Autodesk Inventor part; units mm, degrees
ref_plane "YZ Plane" through (0, 0, 0) normal (1, 0, 0) x (0, 1, 0)
ref_plane "XZ Plane" through (0, 0, 0) normal (0, 1, 0) x (-1, 0, 0)
ref_plane "XY Plane" through (0, 0, 0) normal (0, 0, 1) x (1, 0, 0)
sketch "Sketch1" plane through (0, 0, 0) normal (0, 0, 1) x (1, 0, 0)
  circle A0 centre (0, 0) radius 19.685
  dimension "d0" = 39.37
extrude "Extrusion1" add sketch "Sketch1" along normal blind 43.815
sketch "Sketch2" plane through (0, 0, 43.815) normal (0, 0, 1) x (1, 0, 0)
  circle A0 centre (0, 0) radius 19.685
  circle A1 centre (0, 0) radius 26.035
  dimension "d4" = 52.07
extrude "Extrusion2" add sketch "Sketch2" along normal blind 1.27 contours A0 | A1
fillet "Fillet1" radius 3.175 2 edges at (-19.685, 0, 0) (-19.685, 0, 43.815)
sketch "Sketch3" plane through (0, 0, 0) normal (0, 0, -1) x (-1, 0, 0)
  circle A0 centre (0, 0) radius 16.51
  circle A1 centre (0, 0) radius 3.175
  dimension "d9" = 6.35
extrude "Extrusion3" cut sketch "Sketch3" against normal blind 2.54 contours A1
properties part number "Lg Motor Top" material "ABS Plastic"
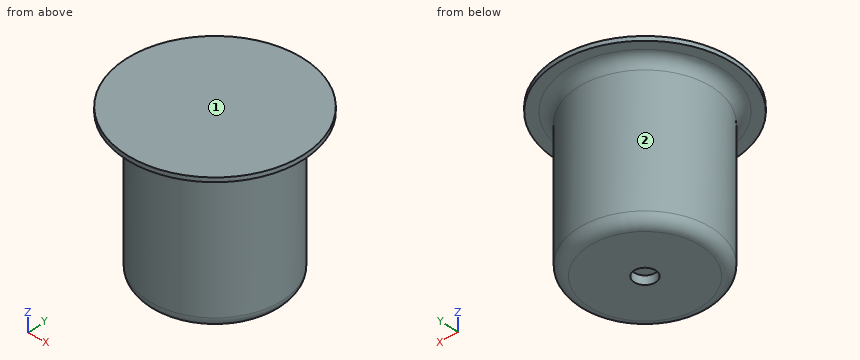
For this review, take the finished solid that the model builds, in its own axes (mm). Face numbers are marked on the shaded views. A direction names the side the tool comes from. Round coordinates to 2 decimals unless told otherwise and drop trailing zeros. Write each loop counter-clockwise with the first axis right and the second up, starting at its lowest first coordinate (ties: lowest second). Pieces come first, ordered by that corner, then holes. Notation, with made-up numbers: (3, 50) -> (20, 50) arc R30 cw to (20, 85) -> close; hole circle Ø11 at (22.5, 53). An arc over 180 degrees is marked (long way). One line per question, with ' | ' between items. Start each with the question number.
1) Add section A-A (x = 0). Write out the cut boundary in (y, z) (3 decimals).
2) For pin 1 Ø5 at (x, z) = (-0.5, 18.5) entering from -Y (3 decimals); pin 2 Ø10 at (x, y) = (-16.5, -15.5) entering from -Z; pin 3 Ø1 at (y, z) = (16.5, 16) entering from -X, all flat-tipped, find the tip position at first contact; note any pin that passes through.
3) Add section C-C (z = 26). Write out the cut boundary in (x, y) (3 decimals), and give its area (3 significant figures).
4) Machinability: for the marked faces 1 and 2, which of the approach directions +Z, -Z, +X, -X, +Y, -Y give a long, thin tool a straight path to every point of the face, cutting with its end or side? Answer none if there is none.
5) Wall thickness on line 1 along Z through (x, y) = (-20, 13.5) (3 decimals); line 2 along Y through (x, z) = (0, 1) (3 decimals); line 3 along Y through (x, z) = (0, 2) (3 decimals): over which ranges is each line inside the solid? List them lowest first.
Reported:
1) outline: (-26.035, 43.815) -> (-22.86, 43.815) arc R3.175 cw to (-19.685, 40.64) -> (-19.685, 3.175) arc R3.175 ccw to (-16.51, 0) -> (-3.175, 0) -> (-3.175, 2.54) -> (3.175, 2.54) -> (3.175, 0) -> (16.51, 0) arc R3.175 ccw to (19.685, 3.175) -> (19.685, 40.64) arc R3.175 cw to (22.86, 43.815) -> (26.035, 43.815) -> (26.035, 45.085) -> (-26.035, 45.085) -> close
2) pin 1: stops at y = -19.685 | pin 2: stops at z = 0.21 | pin 3: stops at x = -11.47
3) outline: circle Ø39.37 at (0, 0) | area: 1,220 mm²
4) face 1: +Z, +X, -X, +Y, -Y | face 2: -Z
5) line 1: z = 43.815 to 45.085 | line 2: y = -18.823 to -3.175, 3.175 to 18.823 | line 3: y = -19.46 to -3.175, 3.175 to 19.46
